Input: part model. Units: mm. Frame: model coordinates. Face numbers are marked on the shaded views. A direction names the side the tool comes from. Give positions to 0.01 mm unless a question says otherwise; leave off trailing zeros. Write each loop counter-clockwise with the first axis right and the second up, starting at its lowest first coordinate (ties: lowest second). Pieces come first, ordered by that corner, then holes. Notation, with made-up numbers: (-4, 55.5) - (18, 55.5) arc R11 ccw to (18, 76.5) - close; hole circle Ø1 at (83.5, 22.25). An arc over 180 degrees is marked (long way). Answer as a JSON object with one key per item and string values. Group by question number.
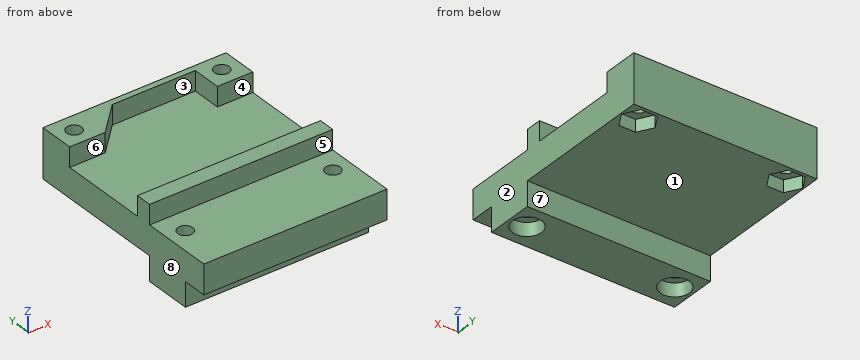
from build123d import *

# Parameters (mm, degrees)
F0_W           = 30
F0_H           = 23.15
F0_H_2         = 6.8
F0_R           = 1.3
F0_H_3         = 4
F0_H_4         = 1
F1_DEPTH       = 12
F2_W           = 5.8
F2_H           = 5.8
F3_DEPTH       = 3.2
F4_DEPTH       = 4
F5_D           = 2.4384
F5_DEPTH       = 10
F5_CBORE_D     = 4.7625
F5_CBORE_DEPTH = 2.1844
F5_TIP         = 0.7325692667
F6_D           = 2.4384
F6_DEPTH       = 20
F6_START       = 4
F6_TIP         = 0.7325692667
F7_DEPTH       = 6


# Not quite as in the source:
# - a feature names something its author has since deleted; it is built from what else it names


with BuildPart() as f1:
    # F0 (on Top) → F1 (new body)
    with BuildSketch(Plane.XY):
        with Locations((0, 23.375)):
            Rectangle(F0_W, F0_H)
        Polygon((-10.7251846715, 34.43125), (-9.350369343, 32.05), (-10.7251846715, 29.66875), (-13.4748153285, 29.66875), (-14.849630657, 32.05), (-13.4748153285, 34.43125), align=None, mode=Mode.SUBTRACT)
        Polygon((10.7251846715, 29.66875), (9.350369343, 32.05), (10.7251846715, 34.43125), (13.4748153285, 34.43125), (14.849630657, 32.05), (13.4748153285, 29.66875), align=None, mode=Mode.SUBTRACT)
        with Locations((0, 7.4)):
            Rectangle(F0_W, F0_H_2)
        with Locations((-12.1, 7.9)):
            Circle(F0_R, mode=Mode.SUBTRACT)
        with Locations((12.1, 7.9)):
            Circle(F0_R, mode=Mode.SUBTRACT)
        with Locations((0, 2)):
            Rectangle(F0_W, F0_H_3)
        with Locations((0, 11.3)):
            Rectangle(F0_W, F0_H_4)
        Polygon((-10.7251846715, 29.66875), (-9.350369343, 32.05), (-10.7251846715, 34.43125), (-13.4748153285, 34.43125), (-14.849630657, 32.05), (-13.4748153285, 29.66875), align=None)
        with Locations((-12.1, 32.05)):
            Circle(F0_R, mode=Mode.SUBTRACT)
        Polygon((10.7251846715, 34.43125), (9.350369343, 32.05), (10.7251846715, 29.66875), (13.4748153285, 29.66875), (14.849630657, 32.05), (13.4748153285, 34.43125), align=None)
        with Locations((12.1, 32.05)):
            Circle(F0_R, mode=Mode.SUBTRACT)
        with Locations((-12.1, 32.05)):
            Circle(F0_R)
        with Locations((12.1, 32.05)):
            Circle(F0_R)
        with Locations((12.1, 7.9)):
            Circle(F0_R)
        with Locations((-12.1, 7.9)):
            Circle(F0_R)
    extrude(amount=F1_DEPTH)

    # F2 (on face) → F3 (cut)
    with BuildSketch(Plane.XY.offset(12)):
        with Locations((-12.1, 7.9)):
            Rectangle(F2_W, F2_H)
        Polygon((9.2, 5), (9.2, 10.8), (-9.2, 10.8), (-9.2, 5), (-15, 5), (-15, 0), (15, 0), (15, 5), align=None)
        with Locations((12.1, 7.9)):
            Rectangle(F2_W, F2_H)
        Polygon((9.2, 10.8), (15, 10.8), (15, 11.8), (-15, 11.8), (-15, 10.8), (-9.2, 10.8), align=None)
        Polygon((-3.4, 14.45), (9.2, 14.45), (9.2, 20.25), (15, 20.25), (15, 29.15), (9.2, 29.15), (9.2, 33.95), (-4.4, 33.95), (-9.2, 29.15), (-13.65, 24.7), (-9.2, 20.25), align=None)
        Polygon((-15, 23.35), (-15, 20.25), (-9.2, 20.25), (-13.65, 24.7), align=None)
        Polygon((-15, 26.05), (-13.65, 24.7), (-9.2, 29.15), (-15, 29.15), align=None)
        Polygon((-15, 26.05), (-15, 23.35), (-13.65, 24.7), align=None)
        Polygon((-9.2, 14.45), (-3.4, 14.45), (-9.2, 20.25), align=None)
        with Locations((-12.1, 17.35)):
            Rectangle(F2_W, F2_H)
        with Locations((12.1, 17.35)):
            Rectangle(F2_W, F2_H)
    extrude(amount=-F3_DEPTH, mode=Mode.SUBTRACT)

    # F0 (on Top) → F4 (cut)
    with BuildSketch(Plane.XY):
        with Locations((0, 23.375)):
            Rectangle(F0_W, F0_H)
        Polygon((-10.7251846715, 34.43125), (-9.350369343, 32.05), (-10.7251846715, 29.66875), (-13.4748153285, 29.66875), (-14.849630657, 32.05), (-13.4748153285, 34.43125), align=None, mode=Mode.SUBTRACT)
        Polygon((10.7251846715, 29.66875), (9.350369343, 32.05), (10.7251846715, 34.43125), (13.4748153285, 34.43125), (14.849630657, 32.05), (13.4748153285, 29.66875), align=None, mode=Mode.SUBTRACT)
        with Locations((0, 2)):
            Rectangle(F0_W, F0_H_3)
        Polygon((-10.7251846715, 29.66875), (-9.350369343, 32.05), (-10.7251846715, 34.43125), (-13.4748153285, 34.43125), (-14.849630657, 32.05), (-13.4748153285, 29.66875), align=None)
        with Locations((-12.1, 32.05)):
            Circle(F0_R, mode=Mode.SUBTRACT)
        Polygon((10.7251846715, 34.43125), (9.350369343, 32.05), (10.7251846715, 29.66875), (13.4748153285, 29.66875), (14.849630657, 32.05), (13.4748153285, 34.43125), align=None)
        with Locations((12.1, 32.05)):
            Circle(F0_R, mode=Mode.SUBTRACT)
        with Locations((-12.1, 32.05)):
            Circle(F0_R)
        with Locations((12.1, 32.05)):
            Circle(F0_R)
    extrude(amount=F4_DEPTH, mode=Mode.SUBTRACT)

    # F5
    with Locations(Plane(origin=(0, 0, 0), x_dir=(1, 0, 0), z_dir=(0, 0, -1))):
        with Locations((-12.1, -7.9), (12.1, -7.9)):
            CounterBoreHole(F5_D / 2, F5_CBORE_D / 2, F5_CBORE_DEPTH, depth=F5_DEPTH)
            with Locations((0, 0, -(F5_DEPTH + F5_TIP / 2))):  # 118° drill point
                Cone(0, F5_D / 2, F5_TIP, mode=Mode.SUBTRACT)

    # F6
    # its depths count from where the whole tool has entered the part; down to there all is cleared
    with Locations(Plane(origin=(0, 0, 0), x_dir=(1, 0, 0), z_dir=(0, 0, -1)).offset(-F6_START)):
        with Locations((-12.1, -32.05), (12.1, -32.05)):
            Hole(F6_D / 2, depth=F6_DEPTH)
            with Locations((0, 0, -(F6_DEPTH + F6_TIP / 2))):  # 118° drill point
                Cone(0, F6_D / 2, F6_TIP, mode=Mode.SUBTRACT)

    # F0 (on Top) → F7 (cut)
    with BuildSketch(Plane.XY):
        Polygon((-10.7251846715, 29.66875), (-9.350369343, 32.05), (-10.7251846715, 34.43125), (-13.4748153285, 34.43125), (-14.849630657, 32.05), (-13.4748153285, 29.66875), align=None)
        with Locations((-12.1, 32.05)):
            Circle(F0_R, mode=Mode.SUBTRACT)
        Polygon((10.7251846715, 34.43125), (9.350369343, 32.05), (10.7251846715, 29.66875), (13.4748153285, 29.66875), (14.849630657, 32.05), (13.4748153285, 34.43125), align=None)
        with Locations((12.1, 32.05)):
            Circle(F0_R, mode=Mode.SUBTRACT)
        with Locations((12.1, 32.05)):
            Circle(F0_R)
        with Locations((-12.1, 32.05)):
            Circle(F0_R)
    extrude(amount=F7_DEPTH, mode=Mode.SUBTRACT)


solid = f1.part
1) Cut plane C-C on z = 8. Return the cut outline in (x, y), and give its area (3 significant figures).
2) Cut plane D-D on y = 7.9. Return the cut outline in (x, z).
3) Mould query, pull axis Y, two halves, no side actions, for the marked faces 6, 7 and 8. Classes: +Y half, -Y half, draft (parallel to the pull), parting line (faces both ways), or undercut.
4) Reachability of the marked faces 1, 2, 3, 4 and 5 from +Z, -Z, +X, -X, +Y, -Y: full face, straight path, thin tool, end or side. Return the list, or none.
5) Cut plane B-B on x = 12.1. Count the separate pieces of the cut face and the enclosed holes in it, and give its area (3 significant figures).
6) Cut plane A-A on z = 11.25. Return the cut outline in (x, y), and give its area (3 significant figures).
7) Pin query (flat end, axial travel): P1, Ø2, axis at x = -12.1, y = 32.05, coming from the +Z side; P2, Ø1, axis at x = -11.5, z = 5, coming from the -Y side; P3, Ø3.5, axis at x = -5, y = 6.5, coming from the +Z side; P4, Ø1.6, axis at x = -10.5, z = 10, coming from the -Y side. Return the tip coordinate at first contact, or that it passes through.
8) Line query: line 1 along Y through (x, z) = (8, 11.5); line 2 along Y through (x, z) = (-12.1, 7.65); line 3 along X through (y, z) = (7.9, 7.5). Output: solid intervals per line, ascending. Write a range as from..to.
Filled in:
{
 "1": {"outline": "(-15, 0) - (15, 0) - (15, 34.95) - (-15, 34.95) - close; hole circle Ø2.44 at (-12.1, 7.9); hole circle Ø2.44 at (-12.1, 32.05); hole circle Ø2.44 at (12.1, 7.9); hole circle Ø2.44 at (12.1, 32.05)", "area": "1,030 mm²"},
 "2": {"outline": "(-15, 0) - (-14.48, 0) - (-14.48, 2.18) - (-13.32, 2.18) - (-13.32, 8.8) - (-15, 8.8) - close; (-10.88, 2.18) - (-9.72, 2.18) - (-9.72, 0) - (9.72, 0) - (9.72, 2.18) - (10.88, 2.18) - (10.88, 8.8) - (-10.88, 8.8) - close; (13.32, 2.18) - (14.48, 2.18) - (14.48, 0) - (15, 0) - (15, 8.8) - (13.32, 8.8) - close"},
 "3": {"face 6": "undercut", "face 7": "+Y half", "face 8": "draft"},
 "4": {"face 1": "-Z, +X, -X, +Y", "face 2": "+Z, -Z, +X, +Y, -Y", "face 3": "+Z", "face 4": "+Z, +X, -X", "face 5": "+Z, +X, -X, -Y"},
 "5": {"separate pieces": "3", "enclosed holes": "0", "area": "175 mm²"},
 "6": {"outline": "(-15, 11.8) - (15, 11.8) - (15, 14.45) - (-15, 14.45) - close; (-15, 29.15) - (-9.2, 29.15) - (-4.4, 33.95) - (9.2, 33.95) - (9.2, 29.15) - (15, 29.15) - (15, 34.95) - (-15, 34.95) - close; hole circle Ø2.44 at (-12.1, 32.05); hole circle Ø2.44 at (12.1, 32.05)", "area": "167 mm²"},
 "7": {"P1": "passes through", "P2": "stops at y = 0", "P3": "stops at z = 8.8", "P4": "stops at y = 11.8"},
 "8": {"line 1": "y = 11.8..14.45, 33.95..34.95", "line 2": "y = 0..6.68, 9.12..30.83, 33.27..34.95", "line 3": "x = -15..-13.32, -10.88..10.88, 13.32..15"}
}
